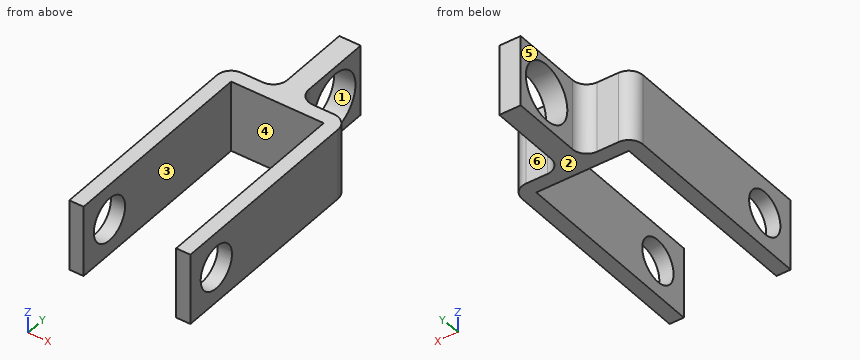
from build123d import *

# Parameters (mm, degrees)
SKETCH1_W               = 10
SKETCH1_H               = 142.4
SKETCH1_H_2             = 10
SKETCH1_W_2             = 25
SKETCH1_W_3             = 15
SKETCH1_H_3             = 60
BOSS_EXTRUDE1_DEPTH     = 50
FILLET1_R               = 10
SKETCH2_R               = 20
CUT_EXTRUDE1_DEPTH      = 36
CUT_EXTRUDE1_DEPTH_BACK = 51
SKETCH3_R               = 15.1
CUT_EXTRUDE2_DEPTH      = 1
CUT_EXTRUDE2_DEPTH_BACK = 86


with BuildPart() as part:
    # Sketch1 → Boss-Extrude1 (new body)
    with BuildSketch(Plane.XY):
        with Locations((-37.5, -106.2)):
            Rectangle(SKETCH1_W, SKETCH1_H)
        with Locations((-37.5, -30)):
            Rectangle(SKETCH1_W, SKETCH1_H_2)
        with Locations((-20, -30)):
            Rectangle(SKETCH1_W_2, SKETCH1_H_2)
        with Locations((0, -30)):
            Rectangle(SKETCH1_W_3, SKETCH1_H_2)
        with Locations((0, 5)):
            Rectangle(SKETCH1_W_3, SKETCH1_H_3)
        with Locations((20, -30)):
            Rectangle(SKETCH1_W_2, SKETCH1_H_2)
        with Locations((37.5, -30)):
            Rectangle(SKETCH1_W, SKETCH1_H_2)
        with Locations((37.5, -106.2)):
            Rectangle(SKETCH1_W, SKETCH1_H)
    extrude(amount=BOSS_EXTRUDE1_DEPTH)

    # Fillet1
    fillet1_edges = [part.edges().sort_by_distance(p)[0] for p in [
        (-42.5, -25, 25),
        (-7.5, -25, 25),
        (7.5, -25, 25),
        (42.5, -25, 25),
    ]]
    fillet(fillet1_edges, radius=FILLET1_R)

    # Sketch2 → Cut-Extrude1 (cut, two sides)
    with BuildSketch(Plane(origin=(7.5, 0, 0), x_dir=(0, 0, -1), z_dir=(1, 0, 0))) as cut_extrude1_sk:
        with Locations((-25, 10)):
            Circle(SKETCH2_R)
    extrude(amount=CUT_EXTRUDE1_DEPTH, mode=Mode.SUBTRACT)
    extrude(cut_extrude1_sk.sketch, amount=-CUT_EXTRUDE1_DEPTH_BACK, mode=Mode.SUBTRACT)

    # Sketch3 → Cut-Extrude2 (cut, two sides)
    with BuildSketch(Plane(origin=(42.5, 0, 0), x_dir=(0, 0, -1), z_dir=(1, 0, 0))) as cut_extrude2_sk:
        with Locations((-25, -152.4)):
            Circle(SKETCH3_R)
    extrude(amount=CUT_EXTRUDE2_DEPTH, mode=Mode.SUBTRACT)
    extrude(cut_extrude2_sk.sketch, amount=-CUT_EXTRUDE2_DEPTH_BACK, mode=Mode.SUBTRACT)


solid = part.part
Work out the finished part from the listing and answer in its coordinate system (mm). Face numbers are marked on the shaded views. A direction names the side the tool comes from. Round coordinates to 2 decimals unless told otherwise and drop trailing zeros. Write each loop counter-clockwise with the first axis right and the second up, starting at its lowest first coordinate (ties: lowest second). Pieces come first, ordered by that corner, then holes. Notation, with made-up numbers: (55, 69.5) -> (87, 69.5) arc R5 ccw to (87, 73.5) -> close; hole circle Ø2 at (2.5, 70). An arc over 180 degrees is marked (long way). Write each question's results on one line, items separated by ' | '.
Item 1: A cutting plane is placed at D-D, the plane x = 11.5. Determine the outline of the cut face in (y, z), plus the area to 3 significant figures.
Result set:
outline: (-35, 0) -> (-23, 0) -> (-23, 50) -> (-35, 50) -> close | area: 600 mm^2
Item 2: Find the intervals of material crossed by line 1 along X through (y, z) = (-90, 29); line 2 along Y through (x, z) = (3, 25); line 3 along Z through (x, y) = (36, -152), in increasing order. Write a range as [from, to].
Result set:
line 1: [-42.5, -32.5], [32.5, 42.5] | line 2: [-35, -10], [30, 35] | line 3: [0, 9.91], [40.09, 50]
Item 3: Which of the six approach directions +Z, -Z, +X, -X, +Y, -Y give full straight-line access (tool end or side, diameter ignored) to the marked faces 4, 5 and 6?
Result set:
face 4: +Z, -Z, -Y | face 5: +Z, -Z, -X, +Y | face 6: +Z, -Z, +X, +Y
Item 4: A cutting plane is placed at A-A, the plane y = -76.5. Determine the outline of the cut face in (x, z).
Result set:
outline: (-42.5, 0) -> (-32.5, 0) -> (-32.5, 50) -> (-42.5, 50) -> close; (32.5, 0) -> (42.5, 0) -> (42.5, 50) -> (32.5, 50) -> close
Item 5: A cutting plane is placed at B-B, the plane z = 25. Determine the outline of the cut face in (x, y), plus the area to 3 significant figures.
Result set:
outline: (-42.5, -177.4) -> (-32.5, -177.4) -> (-32.5, -167.5) -> (-42.5, -167.5) -> close; (-42.5, -137.3) -> (-32.5, -137.3) -> (-32.5, -35) -> (32.5, -35) -> (32.5, -137.3) -> (42.5, -137.3) -> (42.5, -35) arc R10 ccw to (32.5, -25) -> (17.5, -25) arc R10 cw to (7.5, -15) -> (7.5, -10) -> (-7.5, -10) -> (-7.5, -15) arc R10 cw to (-17.5, -25) -> (-32.5, -25) arc R10 ccw to (-42.5, -35) -> close; (-7.5, 30) -> (7.5, 30) -> (7.5, 35) -> (-7.5, 35) -> close; (32.5, -177.4) -> (42.5, -177.4) -> (42.5, -167.5) -> (32.5, -167.5) -> close | area: 3,390 mm^2
Item 6: The mould has two halves that part along Z. Classify the marked faces 1, 2 and 3: +Z half, -Z half, draft (parallel to the pull), parting line (faces both ways), or undercut.
Result set:
face 1: undercut | face 2: -Z half | face 3: draft
Item 7: Flat-ended cylindrical pins translate along their axes: P1, Ø1, axis at y = -3, z = 12.5, coming from the -X side; P2, Ø3, axis at x = 26, z = 41.5, coming from the +Y side; P3, Ø16.5, axis at x = -24.5, z = 13.5, coming from the +Y side; P4, Ø12, axis at x = 33, y = -151.5, coming from the -Z side. Find the tip coordinate at first contact, or state that the pin passes through.
Result set:
P1: through | P2: y = -25 | P3: y = -24.92 | P4: z = 0
Item 8: A cutting plane is placed at C-C, the plane y = -152.4. Determine the outline of the cut face in (x, z), plus the area to 3 significant figures.
Result set:
outline: (-42.5, 0) -> (-32.5, 0) -> (-32.5, 9.9) -> (-42.5, 9.9) -> close; (-42.5, 40.1) -> (-32.5, 40.1) -> (-32.5, 50) -> (-42.5, 50) -> close; (32.5, 0) -> (42.5, 0) -> (42.5, 9.9) -> (32.5, 9.9) -> close; (32.5, 40.1) -> (42.5, 40.1) -> (42.5, 50) -> (32.5, 50) -> close | area: 396 mm^2
